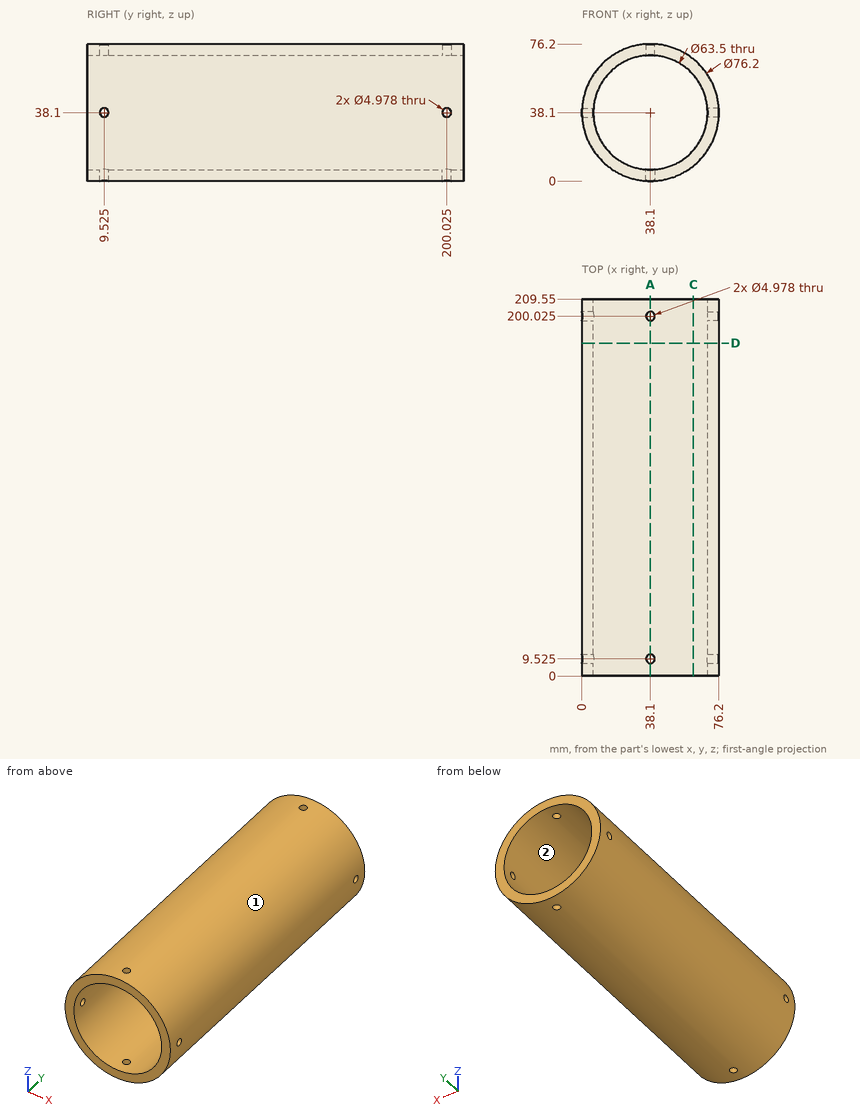
Could you check a few things on this drawing? It's one solid part, dimensions in mm from its lowest x, y, z. Give positions to 0.01 mm unless a question says otherwise; leave off trailing zeros. Order: outer loops, then holes, each group sorted by start corner. A loop starts at its lowest first (then second) coordinate and runs counter-clockwise, first axis right, second up. Notation, with made-up numbers: (22, 29.5) -> (73, 29.5) arc R27 cw to (73, 50.5) -> close; hole circle Ø11 at (86, 22). An arc over 180 degrees is marked (long way). Use CSV: the item, a comma, the result in double quotes. Start each with the question number.
Item 1: Suppose I cut it at D-D (y = 185). List the corners of the cut face in (x, z) for me, and give its area (3 significant figures).
Item 2: If I drill on probe 1 along Y at (x, z) = (5, 38); probe 2 along X at (y, z) = (100.5, 41.5); probe 3 along X at (y, z) = (87, 35.5), over which ranges is the centre line in solid material (lowest first)? Write a range as [from, to].
Item 3: I'm going to push flat-ended pins straight in: P1, Ø1.5, axis at x = 64, z = 9, coming from the +Y side; P2, Ø3, axis at y = 33, z = 30.5, coming from the +X side; P3, Ø6, axis at y = 161.5, z = 17, coming from the +X side; P4, Ø8, axis at y = 147, z = 26.5, coming from the -X side. Where does each tip first touch, or does it pass through?
Item 4: Suppose I cut it at A-A (x = 38.1). Give the number of separate pieces and of enclosed holes in the cut face.
Item 5: Thinking about a two-plate mould opening in X: for the marked faces 1 and 2, which applies, pulls with the +X half, pulls with the -X half, needs draft (parallel to the pull), parting line crosses it, or undercut?
Item 6: Suppose I cut it at C-C (x = 62). List the corners of the cut face in (y, z) for me.
Answer block:
1,outline,"circle Ø76.2 at (38.1, 38.1); hole circle Ø63.5 at (38.1, 38.1)"
1,area,"1,390 mm^2"
2,probe 1,"y = [0, 7.04], [12.01, 197.54], [202.51, 209.55]"
2,probe 2,"x = [0.15, 6.53], [69.67, 76.05]"
2,probe 3,"x = [0.09, 6.46], [69.74, 76.11]"
3,P1,"passes through"
3,P2,"stops at x = 75.71"
3,P3,"stops at x = 71.63"
3,P4,"stops at x = 0.77"
4,separate pieces,"6"
4,enclosed holes,"0"
5,face 1,"parting line crosses it"
5,face 2,"undercut"
6,outline,"(0, 8.43) -> (209.55, 8.43) -> (209.55, 17.2) -> (0, 17.2) -> close; (0, 59) -> (209.55, 59) -> (209.55, 67.77) -> (0, 67.77) -> close"
